Design review of the part shown in the three views and the two pictorial views. Dimensions are in mm from the part's minimum x, y and z. A direction names the side the tool comes from. Round coordinates to 2 decimals unless told otherwise and drop trailing zeros. Order: outer loops, then holes, each group sorted by start corner. A loop starts at its lowest first (then second) coordinate and runs counter-clockwise, first axis right, second up. Notation, with made-up numbers: (8, -2) - (36, -2) arc R20 cw to (36, 33) - close; hole circle Ø3 at (67, -3.75). An arc over 180 degrees is marked (long way). One line per question, with ' | ' between items. Start each with the question number.
Item 1: Add section C-C on z = 69. State the section outline as (x, y) points (1 decimal).
Item 2: Add section A-A on y = 53. State the section outline as (x, z) points.
Item 3: For L1, parallel to Z at x = 45, y = 4; L2, parallel to X at y = 54.5, z = 45.5; L3, parallel to X at y = 62, z = 76, list the stretches that pass through material, from the lowest coordinate up. Write a range as [from, to].
Item 4: Insertion check: pin 1 Ø10 at (x, y) = (36.5, 55.5) entering from +Z; pin 2 Ø5 at (x, z) = (10, 26) entering from +Y. Each pin has a flat end and moves straight along its axis. Give the tip position at first contact, or say it passes through.
Item 5: Tool access review of the marked faces 1 and 2: name each direction out of +Z, -Z, +X, -X, +Y, -Y from which nothing blocks a thin tool from reaching the whole face with its end or side.
Item 6: Add section B-B on x = 39. State the section outline as (y, z) points (1 decimal).
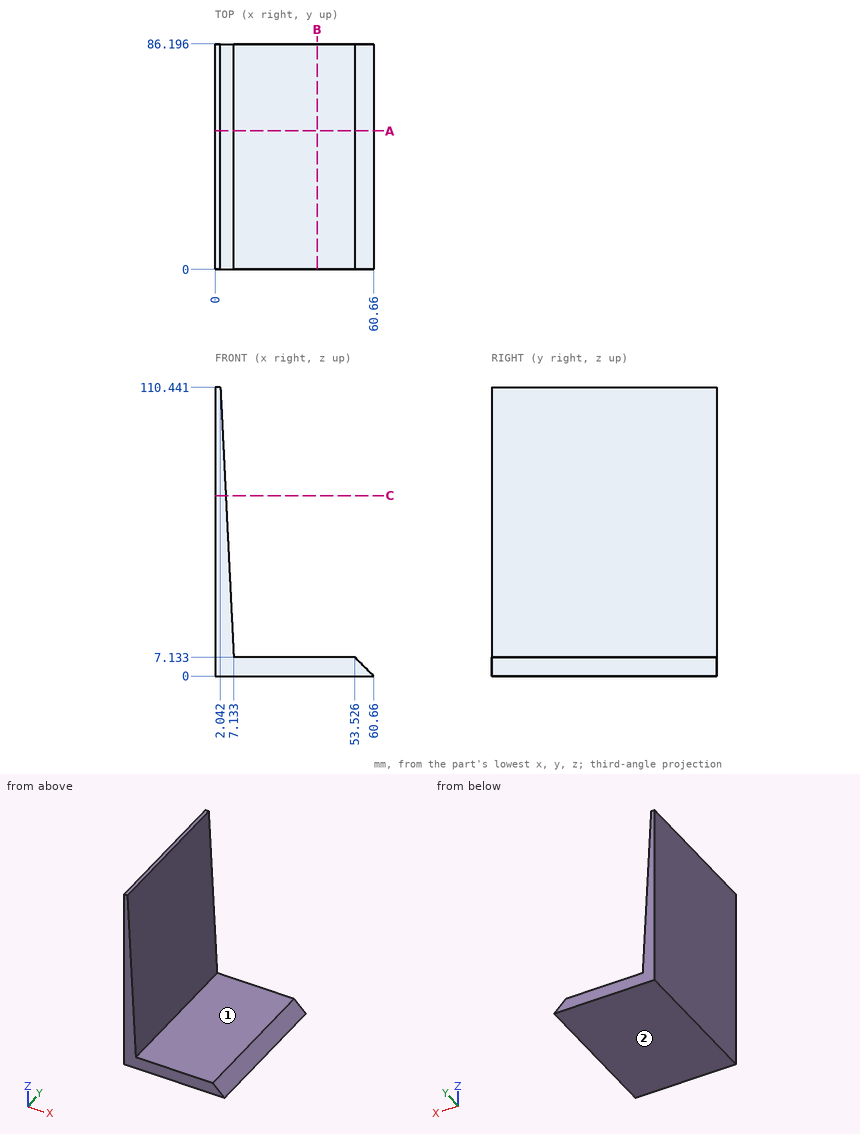
Determined:
1) outline: (0, 0) - (4.1, 0) - (4.1, 86.2) - (0, 86.2) - close
2) outline: (0, 0) - (60.66, 0) - (53.53, 7.13) - (7.13, 7.13) - (2.04, 110.44) - (0, 110.44) - close
3) L1: [0, 7.13] | L2: [0, 5.24] | L3: [0, 3.74]
4) pin 1: z = 7.13 | pin 2: through
5) face 1: +Z, +X, +Y, -Y | face 2: -Z, +X, -X, +Y, -Y
6) outline: (0, 0) - (86.2, 0) - (86.2, 7.1) - (0, 7.1) - close
